Here's how the part is built. I have some questions about the finished solid (model axes, mm). A direction names the side the tool comes from. Coordinates: 2 decimals unless noted, no trailing zeros. Write each loop counter-clockwise with the first axis right and the second up, starting at its lowest first coordinate (ties: lowest second). Pieces come first, ordered by that corner, then holes.
(1) Imagine slicing it at A-A, the plane z = 28. List the corners of the cut face in (x, y) for me.
(2) Which directions (+Z, -Z, +X, -X, +Y, -Y) give clear straight access to the entire face, cutting with the end or side of a thin tool? Please do faces 1 (the flat face through (-512.073, -329.129, 4.004)), 2 (the flat face through (-13, 0, 4)).
(3) For pin 1 Ø5 at (y, z) = (-204.5, 230) entering from +X; pin 2 Ø5 at (y, z) = (-239, 100) entering from +X; pin 3 Ø1.5 at (y, z) = (-361.5, 155) entering from -X, each with a flat end and sliding along its axis, tell me the tip position at first contact or that it passes through.
(4) Please list where these lines run through material, in increasing order: probe 1 along Y at (x, z) = (-173, 165); probe 2 along X at (y, z) = (-271, 25); probe 3 along X at (y, z) = (-21.5, 225).
(5) Imagine slicing it at B-B, the plane x = 48. List the corners of the cut face in (y, z) for me.
```python
from build123d import *

# Parameters (mm, degrees)
BOSS_EXTRUDE1_DEPTH = 296
FILLET1_R           = 10


with BuildPart() as part:
    # Sketch1 → Boss-Extrude1 (new, symmetric)
    with BuildSketch(Plane.XY):
        with BuildLine():
            Line((-225, 75), (-225, 0))
            ThreePointArc((-225, 0), (-321.184305783, -32.650172234), (-377.616280554, -117.106590874))
            Line((-377.616280554, -117.106590874), (-450.060717525, -97.695162491))
            ThreePointArc((-450.060717525, -97.695162491), (-366.841412959, 26.851328288), (-225, 75))
        make_face()
        Polygon((167.450475902, 75), (-225, 75), (-225, 0), (225, 0), align=None)
        Polygon((-578.434963896, -576.79437233), (-505.990526925, -596.205800713), (-377.616280554, -117.106590874), (-450.060717525, -97.695162491), align=None)
    extrude(amount=BOSS_EXTRUDE1_DEPTH, both=True)

    # Fillet1
    fillet1_edges = [part.edges().sort_by_distance(p)[0] for p in [
        (0, 0, 296),
        (-542.21274541, -586.500086522, -296),
        (-514.247840711, -337.244767411, -296),
        (-366.841412959, 26.851328288, -296),
        (-28.774762049, 75, -296),
        (196.225237951, 37.5, -296),
        (0, 0, -296),
        (-321.184305783, -32.650172234, -296),
        (196.225237951, 37.5, 296),
        (-505.990526925, -596.205800713, 0),
        (-578.434963896, -576.79437233, 0),
        (167.450475902, 75, 0),
        (225, 0, 0),
        (-28.774762049, 75, 296),
        (-366.841412959, 26.851328288, 296),
        (-514.247840711, -337.244767411, 296),
        (-542.21274541, -586.500086522, 296),
        (-441.803403739, -356.656195793, 296),
        (-321.184305783, -32.650172234, 296),
        (-441.803403739, -356.656195793, -296),
    ]]
    fillet(fillet1_edges, radius=FILLET1_R)


solid = part.part
```
Recorded:
1. outline: (-575.85, -567.14) arc R10 ccw to (-568.78, -579.38) - (-515.65, -593.62) arc R10 ccw to (-503.4, -586.55) - (-377.62, -117.11) arc R158 cw to (-225, 0) - (204.72, 0) arc R10 ccw to (212.66, 16.09) - (170.45, 71.09) arc R10 ccw to (162.52, 75) - (-225, 75) arc R233 ccw to (-450.06, -97.7) - close
2. face 1: +Z, -Z, -X, +Y
2. face 2: +Z, -Z, +X, -Y
3. pin 1: stops at x = -400.36
3. pin 2: stops at x = -409.61
3. pin 3: stops at x = -520.95
4. probe 1: y = 0 to 75
4. probe 2: x = -496.5 to -418.85
4. probe 3: x = -413.83 to -304.57
5. outline: (0, -286) arc R10 ccw to (10, -296) - (65, -296) arc R10 ccw to (75, -286) - (75, 286) arc R10 ccw to (65, 296) - (10, 296) arc R10 ccw to (0, 286) - close
